Source: CAD feature listing. Evaluate the final solid. Frame: model axes, mm. A direction names the side the tool comes from. Give positions to 0.01 mm unless a question says otherwise; leave off trailing zeros. Loops run counter-clockwise (first coordinate to the right, second up) from the corner with the lowest first, then second, coordinate; pieces in that order, holes last. Notation, with made-up numbers: (66, 21.25) -> (96, 21.25) arc R16 ccw to (96, 41.25) -> close; hole circle Ø2 at (-38.75, 46.25). An arc over 180 degrees is marked (long way). Answer as a JSON object with one key per item and string values. Group by question number.
from build123d import *

# Parameters (mm, degrees)
PAD014_DEPTH           = 2
SKETCH024_R            = 1.375
PAD011_DEPTH           = 6
CUT045_PLACEMENT_ANGLE = 180


with BuildPart() as slotscrew001:
    # Sketch027 → Pad014 (new body)
    with BuildSketch(Plane.XZ):
        with BuildLine():
            ThreePointArc((8.9, 35), (5.9, 38), (2.9, 35))
            Line((2.9, 35), (2.9, 13))
            ThreePointArc((2.9, 13), (5.9, 10), (8.9, 13))
            Line((8.9, 13), (8.9, 35))
        make_face()
    extrude(amount=PAD014_DEPTH)


with BuildPart() as slotscrew001_1:
    # Body013 placement: moved
    add(slotscrew001.part.moved(Location((-0.013, -4.05, -39.977))))


with BuildPart() as base001:
    # Sketch024 → Pad011 (new body)
    with BuildSketch(Plane.XZ):
        with BuildLine():
            Line((-4, 0), (10, 0))
            Line((10, 0), (10, -30.2))
            ThreePointArc((8.2, -32), (9.472792, -31.472792), (10, -30.2))
            Line((8.2, -32), (-2.2, -32))
            ThreePointArc((-4, -30.2), (-3.472792, -31.472792), (-2.2, -32))
            Line((-4, -30.2), (-4, 0))
        make_face()
        with Locations((-1.9, -15.9)):
            Circle(SKETCH024_R, mode=Mode.SUBTRACT)
        with BuildLine():
            ThreePointArc((4.4, -26.9), (5.9, -28.4), (7.4, -26.9))
            Line((7.4, -26.9), (7.4, -4.9))
            ThreePointArc((7.4, -4.9), (5.9, -3.4), (4.4, -4.9))
            Line((4.4, -4.9), (4.4, -26.9))
        make_face(mode=Mode.SUBTRACT)
    extrude(amount=PAD011_DEPTH)

    # Cut045: cut slotscrew001
    add(slotscrew001_1.part, mode=Mode.SUBTRACT)


with BuildPart() as base001_1:
    # Cut045 placement: moved
    add(base001.part.moved(Location((0, 0.008, 7.997))).rotate(Axis((0, 0.008, 7.997), (1, 0, 0)), CUT045_PLACEMENT_ANGLE))


solid = base001_1.part
(1) Section query D-D on y = 0.5. Return the cut outline in (x, z) (3 decimals), plus the area to 3 significant figures.
(2) Material intervals for line 1 (Z direction, x = -1.9, y = 1.7); line 2 (X direction, y = 0.75, z = 16); line 3 (X direction, y = 5.25, z = 28), sorted ascending. Write a range as from..to.
(3) Section query C-C on z = 23. Return the cut outline in (x, y), plus the area to 3 significant figures.
(4) Section query B-B on x = -1.9. Return the cut outline in (y, z).
(5) Mould query, pull axis X, two halves, no side actions, for faces 1 (the face through (-2.079, 2.966, 22.534)), 2 (the face through (9.46, 2.97, 39.48)), 3 (the face through (3, 0.008, 24)), 4 (the face through (-3.487, 2.966, 39.456)). Classes: pulls with the +X half, pulls with the -X half, needs draft (parallel to the pull), parting line crosses it, or undercut.
(6) Section query A-A on z = 17. Return the cut outline in (x, y), plus the area to 4 significant figures.
(7) Access query for faces 5 (the face through (5.953, 5.019, 9.975)), 6 (the face through (2, 6.008, 24)), 7 (the face through (4.4, 2, 24)). Directions: +Z, -Z, +X, -X, +Y, -Y. A direction counts if a zero-diameter tool reaches every point of the face in a straight line with its end or side. Return the directions, or none.
Result:
{
 "1": {"outline": "(-4, 7.997) -> (10, 7.997) -> (10, 38.197) arc R1.8 ccw to (8.2, 39.997) -> (-2.2, 39.997) arc R1.8 ccw to (-4, 38.197) -> close; hole circle Ø2.75 at (-1.9, 23.897); hole (4.4, 12.897) arc R1.5 ccw to (7.4, 12.897) -> (7.4, 34.897) arc R1.5 ccw to (4.4, 34.897) -> close", "area": "368 mm²"},
 "2": {"line 1": "8..22.52, 25.27..40", "line 2": "-4..4.4, 7.4..10", "line 3": "-4..2.89, 8.89..10"},
 "3": {"outline": "(-4, 0.01) -> (-2.94, 0.01) -> (-2.94, 6.01) -> (-4, 6.01) -> close; (-0.86, 0.01) -> (4.4, 0.01) -> (4.4, 4.06) -> (2.89, 4.06) -> (2.89, 6.01) -> (-0.86, 6.01) -> close; (7.4, 0.01) -> (10, 0.01) -> (10, 6.01) -> (8.89, 6.01) -> (8.89, 4.06) -> (7.4, 4.06) -> close", "area": "47.6 mm²"},
 "4": {"outline": "(0.01, 8) -> (6.01, 8) -> (6.01, 22.52) -> (0.01, 22.52) -> close; (0.01, 25.27) -> (6.01, 25.27) -> (6.01, 40) -> (0.01, 40) -> close"},
 "5": {"face 1": "undercut", "face 2": "pulls with the +X half", "face 3": "needs draft", "face 4": "pulls with the -X half"},
 "6": {"outline": "(-4, 0.01) -> (4.4, 0.01) -> (4.4, 4.06) -> (2.89, 4.06) -> (2.89, 6.01) -> (-4, 6.01) -> close; (7.4, 0.01) -> (10, 0.01) -> (10, 6.01) -> (8.89, 6.01) -> (8.89, 4.06) -> (7.4, 4.06) -> close", "area": "60.15 mm²"},
 "7": {"face 5": "+Y", "face 6": "+Z, -Z, +X, -X, +Y", "face 7": "+Y, -Y"}
}
